Design review of the part shown in the three views and the two pictorial views. Dimensions are in mm from the part's minimum x, y and z. A direction names the side the tool comes from. Coordinates: 2 decimals unless noted, no trailing zeros. Write each loop counter-clockwise with the first axis right and the second up, starting at its lowest first coordinate (ties: lowest second). Pieces come first, ordered by that corner, then holes. Notation, with made-up numbers: M 29.5,40.5 L 69.5,40.5 A27 ccw 69.5,73.5 Z; hole C -18.75,64.5 d3. An arc over 180 degrees is marked long. Answer as a JSON object with one key per item and string values.
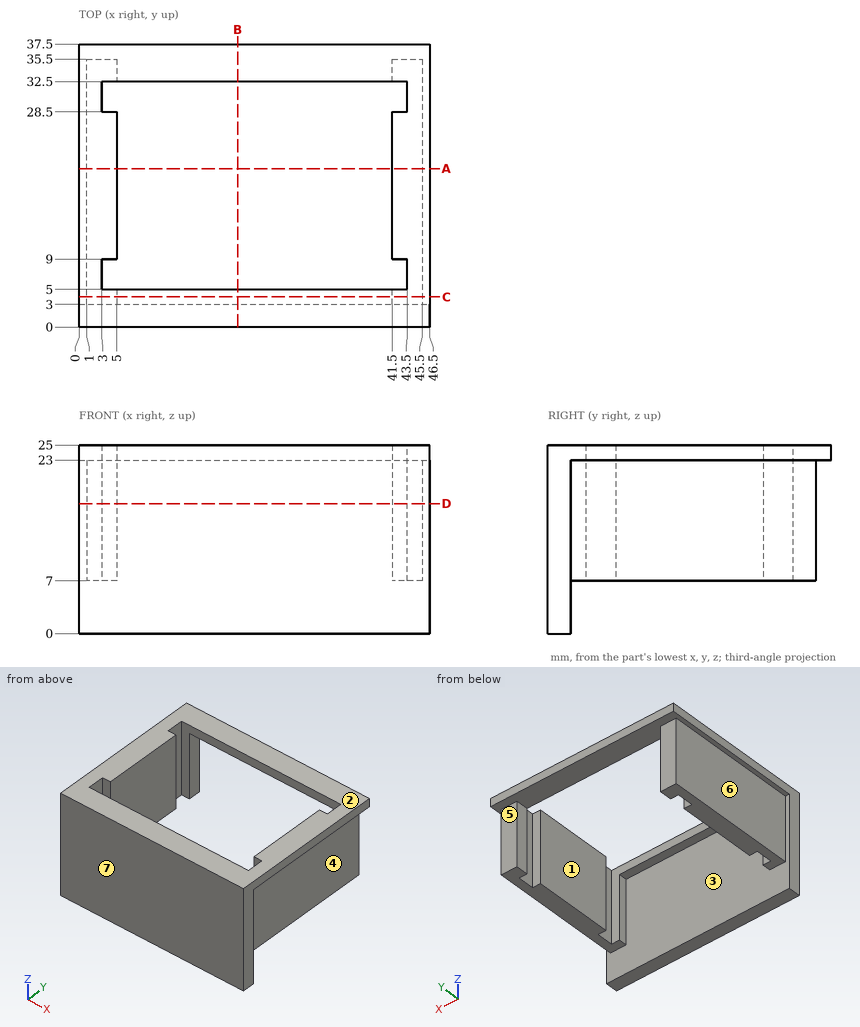
(1) Add section B-B on x = 21. Give the boundary of the cut face in (y, z), and give its area (3 significant figures).
Results list:
{"outline": "M 0,0 L 3,0 L 3,23 L 5,23 L 5,25 L 0,25 Z; M 32.5,23 L 37.5,23 L 37.5,25 L 32.5,25 Z", "area": "89.0 mm²"}
(2) For the marked faces 5, 6 and 7, list the 3-axis set-ups (+Z, -Z, +X, -X, +Y, -Y) from which the entire face can be reached by the end or side of a thin tool; tool diameter is ignored.
Results list:
{"face 5": "-Z, +X, -X, +Y", "face 6": "-Z, -X, +Y", "face 7": "+Z, -Z, +X, -X, -Y"}
(3) For pin 1 Ø1.2 at (x, z) = (44, 15.5) entering from +Y; pin 2 Ø1.5 at (y, z) = (21.5, 20) entering from -X; pin 3 Ø4 at (y, z) = (27.5, 4.5) entering from +X; pin 4 Ø8 at (y, z) = (18, 12.5) entering from +X, all flat-tipped, find the tip position at first contact; note any pin that passes through.
Results list:
{"pin 1": "y = 35.5", "pin 2": "x = 1", "pin 3": "through", "pin 4": "x = 45.5"}
(4) Add section C-C on y = 4. Give the boundary of the cut face in (x, z), and give its area (3 significant figures).
Results list:
{"outline": "M 0,23 L 1,23 L 1,7 L 5,7 L 5,23 L 41.5,23 L 41.5,7 L 45.5,7 L 45.5,23 L 46.5,23 L 46.5,25 L 0,25 Z", "area": "221 mm²"}
(5) Add section D-D on z = 17.25. Give the boundary of the cut face in (x, y).
Results list:
{"outline": "M 0,0 L 46.5,0 L 46.5,3 L 45.5,3 L 45.5,35.5 L 41.5,35.5 L 41.5,32.5 L 43.5,32.5 L 43.5,28.5 L 41.5,28.5 L 41.5,9 L 43.5,9 L 43.5,5 L 41.5,5 L 41.5,3 L 5,3 L 5,5 L 3,5 L 3,9 L 5,9 L 5,28.5 L 3,28.5 L 3,32.5 L 5,32.5 L 5,35.5 L 1,35.5 L 1,3 L 0,3 Z"}
(6) Wall thickness on line 1 along X through (y, z) = (6, 8.25); line 2 along X through (y, z) = (24.5, 22); line 3 along Y through (x, z) = (33.5, 17): over which ranges is each line inside the solid? List them lowest first. Write a range as from..to.
Results list:
{"line 1": "1..3, 43.5..45.5", "line 2": "1..5, 41.5..45.5", "line 3": "0..3"}
(7) Add section A-A on y = 21. Give the boundary of the cut face in (x, z), and give its area (3 significant figures).
Results list:
{"outline": "M 0,23 L 1,23 L 1,7 L 5,7 L 5,25 L 0,25 Z; M 41.5,7 L 45.5,7 L 45.5,23 L 46.5,23 L 46.5,25 L 41.5,25 Z", "area": "148 mm²"}
(8) Draft analysis for pull direction X (two halves, no side actions). For the marked faces 1, 2, 3 and 4, state which applies: released by +X, released by -X, zero draft, split by the parting line, or undercut.
Results list:
{"face 1": "undercut", "face 2": "zero draft", "face 3": "undercut", "face 4": "released by +X"}
